Read the model definition and answer for the solid it produces. Units are mm, in the model's axes. A direction names the side the tool comes from. Round coordinates to 2 decimals unless told otherwise and drop trailing zeros. Order: outer loops, then holes, each group sorted by start corner. A loop starts at its lowest first (then second) coordinate and runs counter-clockwise, first axis right, second up. Notation, with made-up numbers: (43.5, 62) -> (90.5, 62) arc R6 ccw to (90.5, 70) -> close; hole circle Ø1 at (56, -21.5). An arc over 180 degrees is marked (long way). One line per item, written item: value. Start each with the question number.
1. Consider line 1 (Y direction, x = 0, z = 22); line 2 (X direction, y = -3, z = 64); line 3 (Z direction, x = 26, y = -13). Determine where each line is inside the solid, lowest interval first.
2. The mould has two halves that part along Y. Classify faces 1 (the face through (50, -25, 12)), 2 (the face through (1, -30, 12)), 3 (the face through (35, -10, 12)), 4 (the face through (-7, -8, 60)): released by +Y, released by -Y, zero draft, split by the parting line, or undercut.
3. Section B-B (x = 12) is taken. Give the vertices of the cut face in (y, z), then the cut area to 3 significant figures.
4. Section A-A (z = 13) is taken. Give the vertices of the cut face in (x, y).
5. Section D-D (z = 73.5) is taken. Give the vertices of the cut face in (x, y).
6. Section C-C (y = -11) is taken. Give the vertices of the cut face in (x, z).
7. Flat-ended cylindrical pins translate along their axes: pin 1 Ø4 at (x, z) = (9.5, 62.5) entering from -Y; pin 2 Ø5 at (x, z) = (23, 47.5) entering from +Y (3 decimals); pin 3 Ø6 at (y, z) = (1, 61.5) entering from -X; pin 4 Ø2 at (x, z) = (-9.5, 52.5) entering from -Y. Find the tip coordinate at first contact, or state that the pin passes through.
8. For faces 5 (the face through (7, 8, 60)), 6 (the face through (-45, -20, 12)), 7 (the face through (45, 20, 12)), 8 (the face through (9, -9, 80)), determine the directions among +Z, -Z, +X, -X, +Y, -Y from which every point of the face is accessible in a straight line to the end or side of a thin tool.
from build123d import *

# Parameters (mm, degrees)
EXTRUDE_1_DEPTH     = 25
SKETCH_2_R          = 20
EXTRUDE_2_DEPTH     = 55
CUT_EXTRUDE_1_DEPTH = 40
SKETCH_4_R          = 8
CUT_EXTRUDE_2_DEPTH = 40


with BuildPart() as part:
    # Эскиз1 → Бобышка-Вытянуть1 (new body)
    with BuildSketch(Plane.XY):
        Polygon((50, -30), (-50, -30), (-50, -20), (-40, -20), (-30, 0), (-40, 20), (-50, 20), (-50, 30), (50, 30), (50, 20), (40, 20), (30, 0), (40, -20), (50, -20), align=None)
    extrude(amount=EXTRUDE_1_DEPTH)

    # Эскиз2 → Бобышка-Вытянуть2 (add)
    with BuildSketch(Plane.XY.offset(25)):
        Circle(SKETCH_2_R)
    extrude(amount=EXTRUDE_2_DEPTH)

    # Эскиз3 → Вырез-Вытянуть1 (cut)
    with BuildSketch(Plane.XY.offset(80)):
        Polygon((15, 0), (0, -15), (-15, 0), (0, 15), align=None)
    extrude(amount=-CUT_EXTRUDE_1_DEPTH, mode=Mode.SUBTRACT)

    # Эскиз4 → Вырез-Вытянуть2 (cut)
    with BuildSketch(Plane.XY.offset(40)):
        Circle(SKETCH_4_R)
    extrude(amount=-CUT_EXTRUDE_2_DEPTH, mode=Mode.SUBTRACT)


solid = part.part
Answer:
1. line 1: -30 to -8, 8 to 30
1. line 2: -19.77 to -12, 12 to 19.77
1. line 3: 0 to 25
2. face 1: zero draft
2. face 2: released by -Y
2. face 3: undercut
2. face 4: undercut
3. outline: (-30, 0) -> (30, 0) -> (30, 25) -> (16, 25) -> (16, 80) -> (3, 80) -> (3, 40) -> (-3, 40) -> (-3, 80) -> (-16, 80) -> (-16, 25) -> (-30, 25) -> close
3. area: 3,020 mm^2
4. outline: (-50, -30) -> (50, -30) -> (50, -20) -> (40, -20) -> (30, 0) -> (40, 20) -> (50, 20) -> (50, 30) -> (-50, 30) -> (-50, 20) -> (-40, 20) -> (-30, 0) -> (-40, -20) -> (-50, -20) -> close; hole circle Ø16 at (0, 0)
5. outline: circle Ø40 at (0, 0); hole (-15, 0) -> (0, -15) -> (15, 0) -> (0, 15) -> close
6. outline: (-35.5, 0) -> (35.5, 0) -> (35.5, 25) -> (16.7, 25) -> (16.7, 80) -> (4, 80) -> (4, 40) -> (-4, 40) -> (-4, 80) -> (-16.7, 80) -> (-16.7, 25) -> (-35.5, 25) -> close
7. pin 1: y = -18.54
7. pin 2: through
7. pin 3: x = -20
7. pin 4: y = -18.1
8. face 5: +Z
8. face 6: +Z, -Z, -X
8. face 7: +Z, -Z, +X
8. face 8: +Z, +X, -X, +Y, -Y
